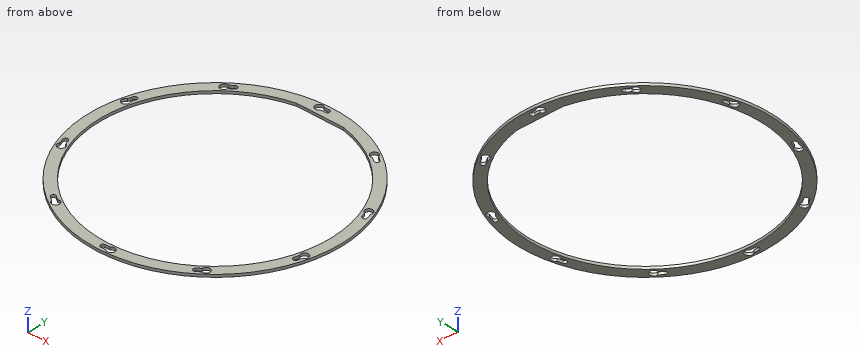
from build123d import *

# Parameters (mm, degrees)
SKETCH1_R            = 191
BOSS_EXTRUDE1_DEPTH  = 4
M6_CLEARANCE_HOLE1_D = 7
CUT_EXTRUDE3_DEPTH   = 5
CIRPATTERN1_COUNT    = 10


with BuildPart() as part:
    # Sketch1 → Boss-Extrude1 (new body)
    with BuildSketch(Plane.XY):
        Circle(SKETCH1_R)
        with BuildLine():
            Line((-35, 171.464281995), (35, 171.464281995))
            ThreePointArc((35, 171.464281995), (0, -175), (-35, 171.464281995))
        make_face(mode=Mode.SUBTRACT)
    extrude(amount=BOSS_EXTRUDE1_DEPTH)

    # M6 Clearance Hole1 (through all)
    with Locations(Plane.XY.offset(4)):
        with Locations((0, 183)):
            m6_clearance_hole1 = Hole(M6_CLEARANCE_HOLE1_D / 2)

    # Sketch4 → Cut-Extrude3 (cut, through all)
    with BuildSketch(Plane.XY.offset(4)):
        with BuildLine():
            Line((0, 186.5), (0, 179.5))
            ThreePointArc((0, 179.5), (-3.626876902, 179.463354933), (-7.252272944, 179.353434696))
            ThreePointArc((-7.252272944, 179.353434696), (-17.735437822, 182.301261264), (-7.623966656, 186.344104099))
            ThreePointArc((-7.623966656, 186.344104099), (-3.81278019, 186.461021952), (0, 186.5))
        make_face()
    cut_extrude3 = extrude(amount=-CUT_EXTRUDE3_DEPTH, mode=Mode.SUBTRACT)

    # CirPattern1: M6 Clearance Hole1, Cut-Extrude3 ×10 about axis
    cirpattern1_axis = Axis((0, 0, 0), (0, 0, 1))
    for i in range(1, CIRPATTERN1_COUNT):
        add(m6_clearance_hole1.rotate(cirpattern1_axis, i * 360 / CIRPATTERN1_COUNT), mode=Mode.SUBTRACT)
        add(cut_extrude3.rotate(cirpattern1_axis, i * 360 / CIRPATTERN1_COUNT), mode=Mode.SUBTRACT)


solid = part.part
Verification items for the finished model (mm, model axes). Coordinates: 2 decimals unless noted, no trailing zeros. Write each loop counter-clockwise with the first axis right and the second up, starting at its lowest first coordinate (ties: lowest second). Pieces come first, ordered by that corner, then holes. Notation, with made-up numbers: M -22,62.5 L -8,62.5 A30 cw -8,86.5 Z; hole C -6.75,54 d8. An arc over 180 degrees is marked long. One line per question, with ' | ' between items.
1) Depth check by flat-ended pin: pin 1 Ø18.5 at (x, y) = (-177.38, 45.02) entering from +Z; pin 2 Ø1 at (y, z) = (31, 1.5) entering from +X; pin 3 Ø1.5 at (x, z) = (-142.5, 1.5) entering from +Y; pin 4 Ø1 at (y, z) = (-105.5, 2.5) entering from +X. Enter the tip coordinate at first touch or a pass-through.
Solutions:
pin 1: z = 4 | pin 2: x = 188.55 | pin 3: y = 128.02 | pin 4: x = 159.55
2) Material ranges on L1, parallel to X at y = 154.5, z = 0.4; L2, parallel to X at y = 65, z = 2.05; L3, parallel to X at y = -53.5, z = 3.7, recorded low to high.
Solutions:
L1: -112.3 to -82.19, 82.19 to 91.89, 104.46 to 112.3 | L2: -179.6 to -162.48, 162.48 to 164.96, 174.97 to 179.6 | L3: -183.35 to -175.76, -172.33 to -166.62, 166.62 to 171.34, 178.66 to 183.35
3) Sectioned sample at B-B on y = 0. Record the cut outline in (x, z).
Solutions:
outline: M -191,0 L -175,0 L -175,4 L -191,4 Z; M 175,0 L 191,0 L 191,4 L 175,4 Z
4) Sectioned sample at A-A on x = -57. Record the cut outline in (y, z).
Solutions:
outline: M -182.3,0 L -165.46,0 L -165.46,4 L -182.3,4 Z; M 165.46,0 L 182.3,0 L 182.3,4 L 165.46,4 Z
5) Sectioned sample at C-C on z = 1.75. State how many separate pieces and enclosed holes the cut face has, then the cut area to 3 significant figures.
Solutions:
separate pieces: 1 | enclosed holes: 11 | area: 16,900 mm^2
